Check sheet for the modelled part. Datum: model origin and axes. Units: mm. Round coordinates to 2 decimals unless told otherwise and drop trailing zeros. Write item = value, one per line.
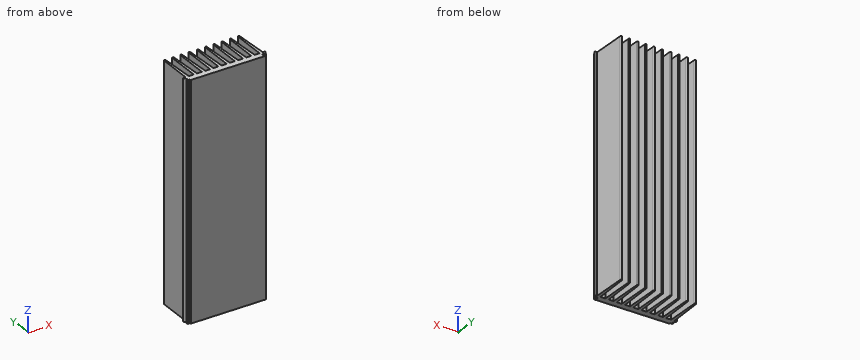
from build123d import *

# Parameters (mm, degrees)
RESSALTO_EXTRUS_O1_DEPTH   = 285
CORTE_EXTRUS_O1_DEPTH      = 1
CORTE_EXTRUS_O1_DEPTH_BACK = 286


with BuildPart() as part:
    # Esboço1 → Ressalto-extrusão1 (new body)
    with BuildSketch(Plane.XY):
        with BuildLine():
            Line((0, 0), (-115.1, 0))
            Line((-115.1, 0), (-115.1, 8))
            Line((-115.1, 8), (-114.1, 49))
            ThreePointArc((-114.1, 49), (-113.1, 50), (-112.1, 49))
            Line((-112.1, 49), (-111.1, 8))
            Line((-111.1, 8), (-105, 8))
            Line((-105, 8), (-104, 49))
            ThreePointArc((-104, 49), (-103, 50), (-102, 49))
            Line((-102, 49), (-101, 8))
            Line((-101, 8), (-94.9, 8))
            Line((-94.9, 8), (-93.9, 49))
            ThreePointArc((-93.9, 49), (-92.9, 50), (-91.9, 49))
            Line((-91.9, 49), (-90.9, 8))
            Line((-90.9, 8), (-84.8, 8))
            Line((-84.8, 8), (-83.8, 49))
            ThreePointArc((-83.8, 49), (-82.8, 50), (-81.8, 49))
            Line((-81.8, 49), (-80.8, 8))
            Line((-80.8, 8), (-74.7, 8))
            Line((-74.7, 8), (-73.7, 49))
            ThreePointArc((-73.7, 49), (-72.7, 50), (-71.7, 49))
            Line((-71.7, 49), (-70.7, 8))
            Line((-70.7, 8), (-64.6, 8))
            Line((-64.6, 8), (-63.6, 49))
            ThreePointArc((-63.6, 49), (-62.6, 50), (-61.6, 49))
            Line((-61.6, 49), (-60.6, 8))
            Line((-60.6, 8), (-54.5, 8))
            Line((-54.5, 8), (-53.5, 49))
            ThreePointArc((-53.5, 49), (-52.5, 50), (-51.5, 49))
            Line((-51.5, 49), (-50.5, 8))
            Line((-50.5, 8), (-44.4, 8))
            Line((-44.4, 8), (-43.4, 49))
            ThreePointArc((-43.4, 49), (-42.4, 50), (-41.4, 49))
            Line((-41.4, 49), (-40.4, 8))
            Line((-40.4, 8), (-34.3, 8))
            Line((-34.3, 8), (-33.3, 49))
            ThreePointArc((-33.3, 49), (-32.3, 50), (-31.3, 49))
            Line((-31.3, 49), (-30.3, 8))
            Line((-30.3, 8), (-24.2, 8))
            Line((-24.2, 8), (-23.2, 49))
            ThreePointArc((-23.2, 49), (-22.2, 50), (-21.2, 49))
            Line((-21.2, 49), (-20.2, 8))
            Line((-20.2, 8), (-14.1, 8))
            Line((-14.1, 8), (-13.1, 49))
            ThreePointArc((-13.1, 49), (-12.1, 50), (-11.1, 49))
            Line((-11.1, 49), (-10.1, 8))
            Line((-10.1, 8), (-4, 8))
            Line((-4, 8), (-3, 49))
            ThreePointArc((-3, 49), (-2, 50), (-1, 49))
            Line((-1, 49), (0, 8))
            Line((0, 8), (0, 0))
        make_face()
    extrude(amount=RESSALTO_EXTRUS_O1_DEPTH)

    # Esboço2 → Corte-extrusão1 (cut, two sides)
    with BuildSketch(Plane.XY.offset(285)) as corte_extrus_o1_sk:
        Polygon((-11.496152423, 0), (0, 0), (0, 52.247610254), (-6.877350269, 52.247610254), (-6.877350269, 8), (-9.496152423, 3.464101615), (-12.527241336, 5.214101615), (-13.527241336, 3.482050808), (-10.496152423, 1.732050808), align=None)
        Polygon((-103.603847577, 0), (-116.981639653, 0), (-116.981639653, 53.433129288), (-108.222649731, 53.433129288), (-108.222649731, 8), (-105.603847577, 3.464101615), (-107.335898385, 2.464101615), (-106.335898385, 0.732050808), (-104.603847577, 1.732050808), align=None)
    extrude(amount=CORTE_EXTRUS_O1_DEPTH, mode=Mode.SUBTRACT)
    extrude(corte_extrus_o1_sk.sketch, amount=-CORTE_EXTRUS_O1_DEPTH_BACK, mode=Mode.SUBTRACT)


solid = part.part
(1) Go/stop test with flat-tipped pins: P1, Ø3, axis at x = -26, z = 182.5, coming from the +Y side; P2, Ø2, axis at x = -55, y = 34.5, coming from the +Z side; P3, Ø2, axis at y = 25.5, z = 177, coming from the -X side; P4, Ø6, axis at y = 42.5, z = 38.5, coming from the -X side. Record where each tip stops, or that it passes through.
Worked answers:
P1 = 8
P2 = through
P3 = -104.6
P4 = -104.23
(2) Sectioned sample at A-A on y = 41. Count the separate pieces of the cut face and the enclosed holes in it, then the cut area to 3 significant figures.
Worked answers:
separate_pieces = 10
enclosed_holes = 0
area = 6,810 mm²
(3) Material ranges on L1, parallel to Y at x = -37, z = 45; L2, parallel to X at y = 5, z = 159; L3, parallel to Y at x = -73, z = 46.5, recorded low to high. Write a range as [from, to].
Worked answers:
L1 = [0, 8]
L2 = [-106.49, -12.65], [-12.16, -8.61]
L3 = [0, 49.95]
